Can you work these out from the model? Positions are in its coordinate system, mm. A direction names the side the tool comes from. Coordinates: 2 decimals unless noted, no trailing zeros. Write each loop counter-clockwise with the first axis right and the second up, starting at its lowest first coordinate (ties: lowest second). Pieces come first, ordered by that corner, then holes. Notation, with made-up numbers: (-12.5, 57) -> (-0.5, 57) arc R21 ccw to (-0.5, 93) -> close; hole circle Ø2 at (-33, 76). An arc over 180 degrees is marked (long way). Answer as CSV lines item,"result". Start each with the question number.
Autodesk Inventor part; units mm, degrees
ref_plane "YZ Plane" through (0, 0, 0) normal (1, 0, 0) x (0, 1, 0)
ref_plane "XZ Plane" through (0, 0, 0) normal (0, 1, 0) x (-1, 0, 0)
ref_plane "XY Plane" through (0, 0, 0) normal (0, 0, 1) x (1, 0, 0)
ref_plane "Work Plane4" through (-12.2663, 62.5, -3) normal (-1, 0, 0) x (0, 0, 1)
sketch "Sketch4" plane through (-12.2663, 62.5, -3) normal (-1, 0, 0) x (0, 0, 1)
  line L0 (0, -23) -> (0, -129)
  line L1 (0, -129) -> (3, -129)
  line L2 (3, -23) -> (3, -129)
  line L3 (0, -23) -> (3, -23)
  circle A0 centre (13.5, 4.5) radius 25
  line L4 (7.5, -146) -> (3, -146)
  line L5 (3, -146) -> (3, -150)
  line L6 (3, -150) -> (-0.5, -150)
  line L7 (-0.5, -150) -> (-0.5, -164)
  line L8 (-0.5, -164) -> (8.5, -150)
  line L9 (8.5, -150) -> (7.5, -150)
  line L10 (7.5, -150) -> (7.5, -146)
  line L11 (0, -132) -> (0, -150)
  line L12 (0, -150) -> (3, -150)
  line L13 (3, -132) -> (3, -150)
  line L14 (3, -107) -> (3, -129)
  line L15 (0, -129) -> (0, -107)
  line L16 (7.5, -146) -> (3, -146)
  line L17 (3, -146) -> (3, -23)
  line L18 (3, -23) -> (36.5, -23)
  line L19 (8.5, -150) -> (66.1149, -60.3768)
  line L20 (7.5, -146) -> (63.7229, -58.5421)
  line L21 (36.5, -23) -> (36.5, -100.8889)
  line L22 (36.5, -98.0889) -> (33.5, -98.0889)
  line L23 (33.5, -98.0889) -> (33.5, -82.9889)
  line L24 (33.5, -82.9889) -> (36.5, -82.9889)
  line L25 (36.5, -82.9889) -> (36.5, -98.0889)
  line L26 (0, -132) -> (3, -132)
  point P0 (3, -62.5)
  point P1 (38.5, 4.5)
  point P2 (3, -129)
  point P3 (3, -132)
  dimension "d4" = 25
  dimension "d5" = 2
  dimension "d9" = 2.8
  dimension "d10" = 15.1
  dimension "d11" = 3
extrude "Extrusion1" add sketch "Sketch4" against normal blind 3 contours L18 L21 L24 L23 L22 L20 L4 L13 L17 L2 | L21 L22 L23 L24
sketch "Sketch10" plane through (-9.2663, 62.5, -3) normal (1, 0, 0) x (0, 0, -1)
  line L0 (-36.5, -23) -> (-36.5, -100.8889)
  line L1 (-36.5, -95.8889) -> (-33, -95.8889)
  line L2 (-33, -95.8889) -> (-33, -80.7889)
  line L3 (-33, -80.7889) -> (-36.5, -80.7889)
  line L4 (-36.5, -80.7889) -> (-36.5, -95.8889)
  point P0 (-3, -62.5)
  point P1 (-36.5, -80.7889)
  dimension "d20" = 3.5
  dimension "d21" = 15.1
  dimension "d22" = 5
extrude "Extrusion4" cut sketch "Sketch10" against normal blind 1.4
ref_plane "Work Plane5" through (1.7337, -83.5, -0.5885) normal (0, 0, 1) x (1, 0, 0)
ref_plane "Work Plane6" through (1.7337, -82.5, 0) normal (0, 0, 1) x (1, 0, 0)
sketch "Sketch13" plane through (1.7337, -82.5, 0) normal (0, 0, 1) x (1, 0, 0)
  circle A0 centre (-5.5, 9.5) radius 1.25
  circle A1 centre (-5.5, 9.5) radius 3
  line L0 (-11, -1) -> (-11, 122)
  line L1 (-11, 12.5) -> (-2.5, 12.5)
  line L2 (-2.5, 12.5) -> (-2.5, 6.5)
  line L3 (-2.5, 6.5) -> (-11, 6.5)
  line L4 (-11, 6.5) -> (-11, 12.5)
  point P0 (-1.7337, 82.5)
  dimension "d28" = 6
extrude "Extrusion6" add sketch "Sketch13" along normal blind 6 contours A0 | A1 | L2 L3 A1 | A1 L1 L2 | A1 L3 L0 L1
sketch "Sketch14" plane through (-9.2663, 62.5, -3) normal (1, 0, 0) x (0, 0, -1)
  line L0 (-3, -23) -> (-36.5, -23)
  line L1 (-36.5, -23) -> (-36.5, -100.8889)
  line L2 (-36.5, -100.8889) -> (-7.5, -146)
  line L3 (-7.5, -146) -> (-3, -146)
  line L4 (-3, -146) -> (-3, -23)
  line L5 (-36.5, -80.7889) -> (-33, -80.7889)
  line L6 (-36.5, -95.8889) -> (-36.5, -80.7889)
  line L7 (-33, -95.8889) -> (-36.5, -95.8889)
  line L8 (-33, -80.7889) -> (-33, -95.8889)
  line L9 (-36.5, -95.8889) -> (-36.5, -100.8889)
  line L10 (-3, -132.5) -> (-3, -23)
  line L11 (-36.5, -95.8889) -> (-3, -95.8889)
  line L12 (-3, -95.8889) -> (-3, -132.5)
  line L13 (-3, -132.5) -> (-36.5, -132.5)
  line L14 (-36.5, -132.5) -> (-36.5, -95.8889)
  line L15 (-3, -138.5) -> (-3, -132.5)
  line L16 (-3, -132.5) -> (-9, -132.5)
  line L17 (-9, -138.5) -> (-9, -132.5)
  line L18 (-3, -138.5) -> (-9, -138.5)
  line L19 (-3, -138.5) -> (-9, -138.5)
  line L20 (-7.5, -146) -> (-36.5, -100.8889)
  line L21 (-9, -138.5) -> (-16.1786, -138.5)
  line L22 (-16.1786, -138.5) -> (-16.1786, -132.5)
  line L23 (-16.1786, -132.5) -> (-9, -132.5)
  line L24 (-9, -132.5) -> (-9, -138.5)
  point P0 (-3, -62.5)
  point P1 (-16.1786, -132.5)
  point P2 (-3, -95.8889)
  point P3 (-12.3214, -138.5)
extrude "Extrusion7" add sketch "Sketch14" along normal blind 4 contours L4 L13 L2 L1 L7 L11 | L17 L21 L2 L13
properties part number "right_side"
Q1. Imagine slicing it at A-A (x = -7.75). Write out the boundary of the cut face in (y, z), then the cut area to 3 significant figures.
Q2. I need wall thicknesses on L1, parallel to Y at x = -2.75, z = 4.5; L2, parallel to Y at x = -5.5, z = 7; L3, parallel to X at y = -21.5, z = 27. Which ranges of each line are inside material? Lowest first, please.
Q3. If we mould it in two halves opening along Y, with no side actions, what happens to faces 4 (the face through (-10.666, -26, 32)), 5 (the face through (-9.266, 4, 17)), 6 (the face through (-5, -76, 4)), 7 (the face through (-3, -70, 3))? For each: released by +Y, released by -Y, zero draft, split by the parting line, or undercut.
Q4. Imagine slicing it at C-C (z = 22). Write out the boundary of the cut face in (x, y).
Q5. Imagine slicing it at D-D (x = -2). Write out the boundary of the cut face in (y, z).
Q6. Imagine slicing it at B-B (y = 6.5). Write out the boundary of the cut face in (x, z).
Q7. For pin 1 (17 mm diameter, centred on y = -56.5, z = 14, fed in from +X); pin 2 (0.7 mm diameter, centred on x = -9.5, y = -27.5, fed in from +Z); pin 3 (1.4 mm diameter, centred on x = -2.5, y = -72, fed in from +Z); pin 4 (4.5 mm diameter, centred on x = -8, z = 19, fed in from +Y), each with a flat end and sliding along its axis, tell me the tip position at first contact or that it passes through.
Q8. Which directions (+Z, -Z, +X, -X, +Y, -Y) give clear straight access to the entire face, cutting with the end or side of a thin tool? Please do faces 1 (the face through (-3, -73, 6)), 2 (the face through (-11, -83.5, 2)), 3 (the face through (-9.266, -80, 4)).
Entries:
1,outline,"(-76, 0) -> (-33.39, 0) -> (-33.39, 33.5) -> (-38.39, 33.5) -> (-76, 9.32) -> close"
1,area,"973 mm2"
2,L1,"-76 to -70"
2,L2,"-76 to -33.39"
2,L3,"-12.27 to -9.27"
3,face 4,"undercut"
3,face 5,"zero draft"
3,face 6,"released by -Y"
3,face 7,"released by +Y"
4,outline,"(-12.27, -56.28) -> (-5.27, -56.28) -> (-5.27, -33.39) -> (-9.27, -33.39) -> (-9.27, 39.5) -> (-12.27, 39.5) -> close"
5,outline,"(-76, 0) -> (-70, 0) -> (-70, 6) -> (-76, 6) -> close"
6,outline,"(-12.27, 0) -> (-9.27, 0) -> (-9.27, 33.5) -> (-12.27, 33.5) -> close"
7,pin 1,"x = -5.27"
7,pin 2,"z = 30"
7,pin 3,"z = 6"
7,pin 4,"y = 39.5"
8,face 1,"+Z, +X, +Y, -Y"
8,face 2,"+Z, -Z, +X, -X, -Y"
8,face 3,"+Z, -Z, +X, -Y"
